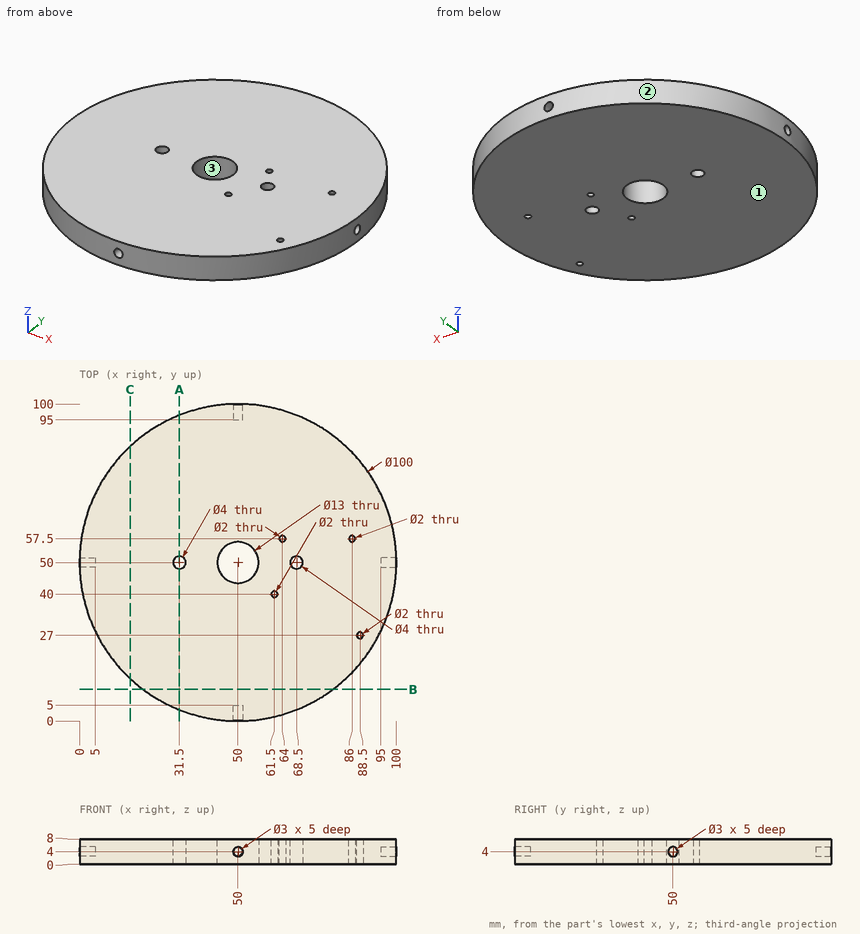
Design review of the part shown in the three views and the two pictorial views. Dimensions are in mm from the part's minimum x, y and z. Coordinates: 2 decimals unless noted, no trailing zeros. Loops run counter-clockwise (first coordinate to the right, second up) from the corner with the lowest first, then second, coordinate; pieces in that order, holes last. Notation, with made-up numbers: M -9.5,71 L 29.5,71 A16 ccw 29.5,101 Z; hole C -0.75,43 d7. An arc over 180 degrees is marked long. One line per question, with ' | ' between items.
(1) We need section C-C (x = 16). Give the boundary of the cut face in (y, z), and give its area (3 significant figures).
Filled in:
outline: M 13.34,0 L 86.66,0 L 86.66,8 L 13.34,8 Z | area: 587 mm^2
(2) For pin 1 Ø2.5 at (y, z) = (50, 4) entering from -X; pin 2 Ø2.5 at (x, y) = (68.5, 50) entering from +Z; pin 3 Ø1.5 at (x, z) = (82.5, 2) entering from -Y; pin 4 Ø4 at (y, z) = (42.5, 5) entering from -X, all flat-tipped, find the tip position at first contact; note any pin that passes through.
Filled in:
pin 1: stops at x = 5 | pin 2: passes through | pin 3: stops at y = 11.37 | pin 4: stops at x = 0.3
(3) Draft analysis for pull direction X (two halves, no side actions). For the marked faces 1, 2 and 3, state which applies: released by +X, released by -X, zero draft, split by the parting line, or undercut.
Filled in:
face 1: zero draft | face 2: split by the parting line | face 3: undercut
(4) We need section B-B (y = 10). Give the boundary of the cut face in (x, z), and give its area (3 significant figures).
Filled in:
outline: M 20,0 L 80,0 L 80,8 L 20,8 Z | area: 480 mm^2
(5) Wall thickness on probe 1 along Y at (x, z) = (50, 3.75); probe 2 along Z at (x, y) = (50, 2.6); probe 3 along X at (y, z) = (45, 3.5): over which ranges is each line inside the solid? List them lowest first.
Filled in:
probe 1: y = 5 to 43.5, 56.5 to 95 | probe 2: z = 0 to 2.5, 5.5 to 8 | probe 3: x = 0.25 to 45.85, 54.15 to 99.75
(6) We need section A-A (x = 31.5). Give the boundary of the cut face in (y, z).
Filled in:
outline: M 3.55,0 L 48,0 L 48,8 L 3.55,8 Z; M 52,0 L 96.45,0 L 96.45,8 L 52,8 Z
